Geometry check sheet. Reference: the model listing, model coordinates, mm. A direction names the side the tool comes from. Round coordinates to 2 decimals unless told otherwise and drop trailing zeros. Loops run counter-clockwise (first coordinate to the right, second up) from the corner with the lowest first, then second, coordinate; pieces in that order, holes last. Notation, with made-up numbers: (88.25, 36) - (115.25, 36) arc R12 ccw to (115.25, 59) - close; hole circle Ø11 at (50, -4). An arc over 180 degrees is marked (long way). Write item = value, one per line.
```python
from build123d import *

# Parameters (mm, degrees)
EXTRUDE_1_DEPTH   = 2
HOLE_WIZARD_M51_D = 5.5
CHAMFER_1_SIZE    = 2


with BuildPart() as part:
    # Эскиз1 → Бобышка-Вытянуть1 (new body)
    with BuildSketch(Plane(origin=(0, 0, 0), x_dir=(1, 0, 0), z_dir=(0, 0, -1))):
        Polygon((0, 0), (0, 40), (40, 40), (40, 20), (20, 20), (20, 0), align=None)
    extrude(amount=EXTRUDE_1_DEPTH)

    # Отверстие с зазором M51 (through all)
    with Locations(Plane(origin=(0, 0, -2), x_dir=(1, 0, 0), z_dir=(0, 0, -1))):
        with Locations((10, 30), (10, 10), (30, 30)):
            Hole(HOLE_WIZARD_M51_D / 2)

    # Фаска1
    chamfer_1_edges = [part.edges().sort_by_distance(p)[0] for p in [
        (0, 0, -1),
        (0, -40, -1),
        (40, -40, -1),
        (40, -20, -1),
        (20, 0, -1),
    ]]
    chamfer(chamfer_1_edges, length=CHAMFER_1_SIZE)


solid = part.part
```
(1) Section check A-A (y = -10). Enter the section's corners in (x, z), then the cut area to 3 significant figures.
Answers follow:
outline = (0, -2) - (7.25, -2) - (7.25, 0) - (0, 0) - close; (12.75, -2) - (20, -2) - (20, 0) - (12.75, 0) - close
area = 29.0 mm²
(2) Set-up check for faces 4 (the flat face through (20, -11, -1)), 5 (the flat face through (40, -30, -1)): record each of +Z, -Z, +X, -X, +Y, -Y from which the full face is reachable in a straight line by a thin tool's end or side.
Answers follow:
face_4 = +Z, -Z, +X, +Y
face_5 = +Z, -Z, +X, +Y, -Y
(3) Gauge pin test, flat ends, axial feed: pin 1 (3.5 mm diameter, centred on x = 10, y = -30, fed in from +Z); pin 2 (1 mm diameter, centred on y = -13.5, z = -1, fed in from +X). Record the tip position at first contact, or that the pin passes through.
Answers follow:
pin_1 = through
pin_2 = 20
(4) Mould release check, pull along Y, two halves, no side actions. Record for faces 1 (the flat face through (39, -39, -1)), 2 (the cylindrical face through (8.52, -32.32, -0.99)), 3 (the flat face through (16, -25, -2)): pulls with the +Y half, pulls with the -Y half, needs draft (parallel to the pull), parting line crosses it, or undercut.
Answers follow:
face_1 = pulls with the -Y half
face_2 = undercut
face_3 = needs draft
(5) Section check B-B (x = 10). Enter the section's corners in (y, z), then the cut area to 3 significant figures.
Answers follow:
outline = (-40, -2) - (-32.75, -2) - (-32.75, 0) - (-40, 0) - close; (-27.25, -2) - (-12.75, -2) - (-12.75, 0) - (-27.25, 0) - close; (-7.25, -2) - (0, -2) - (0, 0) - (-7.25, 0) - close
area = 58.0 mm²
(6) Section check C-C (y = -30). Enter the section's corners in (x, z).
Answers follow:
outline = (0, -2) - (7.25, -2) - (7.25, 0) - (0, 0) - close; (12.75, -2) - (27.25, -2) - (27.25, 0) - (12.75, 0) - close; (32.75, -2) - (40, -2) - (40, 0) - (32.75, 0) - close
(7) Section check D-D (x = 30). Enter the section's corners in (y, z).
Answers follow:
outline = (-40, -2) - (-32.75, -2) - (-32.75, 0) - (-40, 0) - close; (-27.25, -2) - (-20, -2) - (-20, 0) - (-27.25, 0) - close
(8) Scan lines: L1, parallel to Y at x = 10, z = -1.25; L2, parallel to X at y = -30, z = -0.75; L3, parallel to X at y = -28, z = -1.05. Record each from-to range of solid material in increasing order. Write a range as [from, to].
Answers follow:
L1 = [-40, -32.75], [-27.25, -12.75], [-7.25, 0]
L2 = [0, 7.25], [12.75, 27.25], [32.75, 40]
L3 = [0, 8.11], [11.89, 28.11], [31.89, 40]
